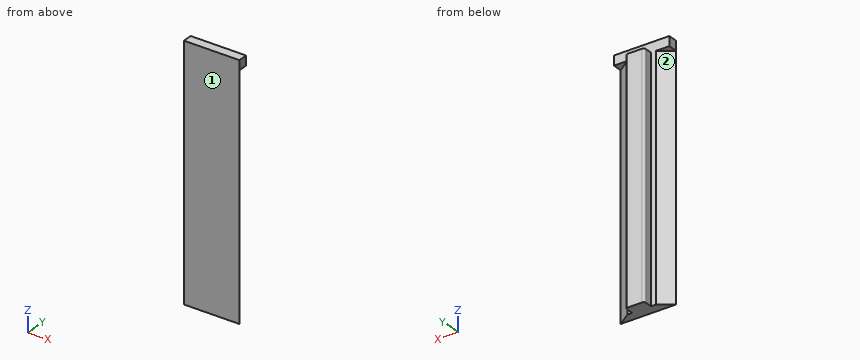
```python
from build123d import *

# Parameters (mm, degrees)
BOSS_EXTRUDE1_DEPTH = 25
SKETCH2_W           = 5.856296014
SKETCH2_H           = 1
BOSS_EXTRUDE2_DEPTH = 1
SKETCH3_W           = 2
SKETCH3_H           = 25
BOSS_EXTRUDE3_DEPTH = 1
FILLET1_R           = 0.25


with BuildPart() as part:
    # Sketch1 → Boss-Extrude1 (new body)
    with BuildSketch(Plane.XY):
        Polygon((0, 0), (-1.428148007, -1), (4.428148007, -1), (3, 0), align=None)
    extrude(amount=BOSS_EXTRUDE1_DEPTH)

    # Sketch2 → Boss-Extrude2 (add)
    with BuildSketch(Plane.XY.offset(25)):
        with Locations((1.5, -0.5)):
            Rectangle(SKETCH2_W, SKETCH2_H)
    extrude(amount=BOSS_EXTRUDE2_DEPTH)

    # Sketch3 → Boss-Extrude3 (add)
    with BuildSketch(Plane(origin=(0, 0, 0), x_dir=(1, 0, 0), z_dir=(0, 1, 0))):
        with Locations((1.5, -12.5)):
            Rectangle(SKETCH3_W, SKETCH3_H)
    extrude(amount=BOSS_EXTRUDE3_DEPTH)

    # Fillet1
    fillet1_edges = [part.edges().sort_by_distance(p)[0] for p in [
        (0.5, 1, 12.5),
        (2.5, 1, 12.5),
    ]]
    fillet(fillet1_edges, radius=FILLET1_R)


solid = part.part
```
Geometry check sheet. Reference: the model listing, model coordinates, mm. Face numbers are marked on the shaded views. A direction names the side the tool comes from. Give positions to 0.01 mm unless a question says otherwise; leave off trailing zeros. Order: outer loops, then holes, each group sorted by start corner. A loop starts at its lowest first (then second) coordinate and runs counter-clockwise, first axis right, second up.
1. Access from +Z, -Z, +X, -X, +Y, -Y to the whole of each face (thin tool, end or side, straight path). Record for the marked faces 1 and 2.
2. Section check B-B, the plane y = -0.6. Enter the section's corners in (x, z).
3. Thickness scan on L1, parallel to Z at x = 4, y = -0.2; L2, parallel to X at y = 0.5, z = 12; L3, parallel to Z at x = 1.45, y = 0.1. Record the ranges inside material, lowest first.
4. Section check A-A, the plane z = 2.75. Enter the section's corners in (x, y), and give its area (3 significant figures).
5. Gauge pin test, flat ends, axial feed: pin 1 Ø0.8 at (y, z) = (0, 14) entering from -X; pin 2 Ø0.8 at (x, y) = (-0.5, -0.5) entering from -Z; pin 3 Ø0.5 at (x, y) = (1.5, 0.5) entering from +Z. Record the tip position at first contact, or that the pin passes through.
6. Section check C-C, the plane x = -0.4. Enter the section's corners in (y, z), and give its area (3 significant figures).
7. Section check D-D, the plane x = 3.35. Enter the section's corners in (y, z), and give its area (3 significant figures).
Values follow:
1. face 1: +Z, -Z, +X, -X, -Y
1. face 2: -Z, -X, +Y
2. outline: (-1.43, 25) - (-0.86, 25) - (-0.86, 0) - (3.86, 0) - (3.86, 25) - (4.43, 25) - (4.43, 26) - (-1.43, 26) - close
3. L1: z = 25 to 26
3. L2: x = 0.5 to 2.5
3. L3: z = 0 to 25
4. outline: (-1.43, -1) - (4.43, -1) - (3, 0) - (2.5, 0) - (2.5, 0.75) arc R0.25 ccw to (2.25, 1) - (0.75, 1) arc R0.25 ccw to (0.5, 0.75) - (0.5, 0) - (0, 0) - close
4. area: 6.40 mm2
5. pin 1: stops at x = -0.57
5. pin 2: stops at z = 0
5. pin 3: stops at z = 25
6. outline: (-1, 0) - (-0.28, 0) - (-0.28, 25) - (0, 25) - (0, 26) - (-1, 26) - close
6. area: 19.0 mm2
7. outline: (-1, 0) - (-0.25, 0) - (-0.25, 25) - (0, 25) - (0, 26) - (-1, 26) - close
7. area: 19.9 mm2
